Design review of the part built by this model. Coordinates are the model's own, in mm. A direction names the side the tool comes from. Coordinates: 2 decimals unless noted, no trailing zeros. Write each loop counter-clockwise with the first axis right and the second up, starting at its lowest first coordinate (ties: lowest second). Pieces come first, ordered by that corner, then holes. Notation, with made-up numbers: (62, 79.5) - (93, 79.5) arc R6 cw to (93, 88.5) - close; hole circle Ø2 at (49, 23). An arc over 180 degrees is marked (long way). Use a Markdown table: item, result.
from build123d import *

# Parameters (mm, degrees)
BOSS_EXTRUDE1_DEPTH  = 12
BOSS_EXTRUDE11_DEPTH = 12
BOSS_EXTRUDE12_DEPTH = 12
BOSS_EXTRUDE13_DEPTH = 12
SKETCH8_R            = 8
CUT_EXTRUDE1_DEPTH   = 128
SKETCH9_R            = 8
CUT_EXTRUDE2_DEPTH   = 128
SKETCH10_R           = 8
CUT_EXTRUDE4_DEPTH   = 128
FILLET4_R            = 3


with BuildPart() as part:
    # Sketch2 → Boss-Extrude1 (new body)
    with BuildSketch(Plane(origin=(0, 0, 0), x_dir=(1, 0, 0), z_dir=(0, 1, 0))):
        with BuildLine():
            Line((-30, 20), (30, 20))
            ThreePointArc((30, 20), (50, 0), (30, -20))
            Line((30, -20), (-30, -20))
            Line((-30, -20), (-30, 20))
        make_face()
    extrude(amount=BOSS_EXTRUDE1_DEPTH)

    # Sketch3 → Boss-Extrude11 (add)
    with BuildSketch(Plane.XY.offset(20)):
        with BuildLine():
            ThreePointArc((10, 32), (-10, 52), (-30, 32))
            Line((-30, 32), (10, 32))
        make_face()
        with BuildLine():
            ThreePointArc((-30, 32), (-24.142135624, 17.857864376), (-10, 12))
            ThreePointArc((-10, 12), (4.142135624, 17.857864376), (10, 32))
            Line((10, 32), (-30, 32))
        make_face()
        with BuildLine():
            Line((-30, 32), (-30, 12))
            Line((-30, 12), (-10, 12))
            ThreePointArc((-10, 12), (-24.142135624, 17.857864376), (-30, 32))
        make_face()
        with BuildLine():
            ThreePointArc((10, 32), (4.142135624, 17.857864376), (-10, 12))
            Line((-10, 12), (10, 12))
            Line((10, 12), (10, 32))
        make_face()
    extrude(amount=-BOSS_EXTRUDE11_DEPTH)

    # Sketch5 → Boss-Extrude12 (add)
    with BuildSketch(Plane(origin=(0, 0, -20), x_dir=(-1, 0, 0), z_dir=(0, 0, -1))):
        with BuildLine():
            Line((10, 12), (30, 12))
            Line((30, 12), (30, 32))
            ThreePointArc((30, 32), (24.142135624, 17.857864376), (10, 12))
        make_face()
        with BuildLine():
            Line((-10, 12), (10, 12))
            ThreePointArc((10, 12), (-4.142135624, 17.857864376), (-10, 32))
            Line((-10, 32), (-10, 12))
        make_face()
        with BuildLine():
            ThreePointArc((-10, 32), (-4.142135624, 17.857864376), (10, 12))
            ThreePointArc((10, 12), (24.142135624, 17.857864376), (30, 32))
            Line((30, 32), (-10, 32))
        make_face()
        with BuildLine():
            Line((-10, 32), (30, 32))
            ThreePointArc((30, 32), (10, 52), (-10, 32))
        make_face()
    extrude(amount=-BOSS_EXTRUDE12_DEPTH)

    # Sketch6 → Boss-Extrude13 (add)
    with BuildSketch(Plane.ZY.offset(30)):
        with BuildLine():
            Line((20, 0), (0, 0))
            ThreePointArc((0, 0), (14.142135624, -5.857864376), (20, -20))
            Line((20, -20), (20, 0))
        make_face()
        with BuildLine():
            Line((0, 0), (-20, 0))
            Line((-20, 0), (-20, -20))
            ThreePointArc((-20, -20), (-14.142135624, -5.857864376), (0, 0))
        make_face()
        with BuildLine():
            ThreePointArc((20, -20), (14.142135624, -5.857864376), (0, 0))
            ThreePointArc((0, 0), (-14.142135624, -5.857864376), (-20, -20))
            Line((-20, -20), (20, -20))
        make_face()
        with BuildLine():
            Line((20, -20), (-20, -20))
            ThreePointArc((-20, -20), (0, -40), (20, -20))
        make_face()
    extrude(amount=-BOSS_EXTRUDE13_DEPTH)

    # Sketch8 → Cut-Extrude1 (cut)
    with BuildSketch(Plane.XY.offset(20)):
        with Locations((-10, 32)):
            Circle(SKETCH8_R)
    extrude(amount=-CUT_EXTRUDE1_DEPTH, mode=Mode.SUBTRACT)

    # Sketch9 → Cut-Extrude2 (cut)
    with BuildSketch(Plane(origin=(0, 12, 0), x_dir=(1, 0, 0), z_dir=(0, 1, 0))):
        with Locations((30.130515164, -0.017591691)):
            Circle(SKETCH9_R)
    extrude(amount=-CUT_EXTRUDE2_DEPTH, mode=Mode.SUBTRACT)

    # Sketch10 → Cut-Extrude4 (cut)
    with BuildSketch(Plane(origin=(-18, 0, 0), x_dir=(0, 0, -1), z_dir=(1, 0, 0))):
        with Locations((0, -20)):
            Circle(SKETCH10_R)
    extrude(amount=-CUT_EXTRUDE4_DEPTH, mode=Mode.SUBTRACT)

    # Fillet4
    fillet4_edges = [part.edges().sort_by_distance(p)[0] for p in [
        (10, 12, 14),
        (-10, 12, 8),
        (10, 12, -14),
        (-10, 12, -8),
        (-18, 0, 0),
    ]]
    fillet(fillet4_edges, radius=FILLET4_R)


solid = part.part
(1) Take a section at D-D on x = 5. Write out the cut boundary in (y, z), and give its area (3 significant figures).
Determined:
| item | result |
|---|---|
| outline | (0, -20) - (45.23, -20) - (45.23, -8) - (15, -8) arc R3 cw to (12, -5) - (12, 5) arc R3 cw to (15, 8) - (45.23, 8) - (45.23, 20) - (0, 20) - close |
| area | 1,280 mm2 |
(2) For pin 1 (3.5 mm diameter, centred on y = 22.5, z = -15.5, fed in from +X); pin 2 (12 mm diameter, centred on x = 19, z = 5.5, fed in from -Y); pin 3 (6 mm diameter, centred on x = -13.5, y = -18, fed in from +Z); pin 4 (12 mm diameter, centred on x = -9, z = -7, fed in from +Y), all flat-tipped, find the tip position at first contact; note any pin that passes through.
Determined:
| item | result |
|---|---|
| pin 1 | x = 10 |
| pin 2 | y = 0 |
| pin 3 | through |
| pin 4 | y = 52 |
(3) Take a section at A-A on z = -17. Write out the cut boundary in (x, y), and give its area (3 significant figures).
Determined:
| item | result |
|---|---|
| outline | (-30, -30.54) - (-18, -30.54) - (-18, -3) arc R3 cw to (-15, 0) - (40.54, 0) - (40.54, 12) - (13, 12) arc R3 cw to (10, 15) - (10, 32) arc R20 ccw to (-30, 32) - close; hole circle Ø16 at (-10, 32) |
| area | 2,440 mm2 |
(4) For L1, parallel to X at y = 9.5, z = 0.5; L2, parallel to Y at x = -10, z = 11; L3, parallel to X at y = 17, z = 17.5, list the stretches that pass through material, from the lowest coordinate up. Write a range as from..to.
Determined:
| item | result |
|---|---|
| L1 | -30..22.15, 38.12..49.99 |
| L2 | 0..24, 40..52 |
| L3 | -30..10 |
(5) Take a section at B-B on y = 26. Write out the cut boundary in (x, z), and give its area (3 significant figures).
Determined:
| item | result |
|---|---|
| outline | (-30, -20) - (-15.29, -20) - (-15.29, -8) - (-30, -8) - close; (-30, 8) - (-15.29, 8) - (-15.29, 20) - (-30, 20) - close; (-4.71, -20) - (10, -20) - (10, -8) - (-4.71, -8) - close; (-4.71, 8) - (10, 8) - (10, 20) - (-4.71, 20) - close |
| area | 706 mm2 |
(6) Draft analysis for pull direction X (two halves, no side actions). For faces 1 (the cylindrical face through (-11.041, 39.932, -13.916)), 2 (the cylindrical face through (-10, 52, 14)), 3 (the flat face through (19, 12, 0)), state which applies: +X half, -X half, draft (parallel to the pull), parting line (faces both ways), or undercut.
Determined:
| item | result |
|---|---|
| face 1 | undercut |
| face 2 | parting line |
| face 3 | draft |
(7) Take a section at C-C on x = -20.5. Write out the cut boundary in (y, z), and give its area (3 significant figures).
Determined:
| item | result |
|---|---|
| outline | (-20, -20) - (49.02, -20) - (49.02, -8) - (15, -8) arc R3 cw to (12, -5) - (12, 5) arc R3 cw to (15, 8) - (49.02, 8) - (49.02, 20) - (-20, 20) arc R20 ccw to start; hole circle Ø16 at (-20, 0) |
| area | 2,600 mm2 |
(8) Machinability: for faces 4 (the flat face through (18, 0, 0)), 5 (the cylindrical face through (37.76, 6.08, -2.39)), 6 (the cylindrical face through (-8.2, 12.86, 7.1)), 7 (the flat face through (10, 23, 14)), which of the approach directions +Z, -Z, +X, -X, +Y, -Y give a long, thin tool a straight path to every point of the face, cutting with its end or side? Answer none if there is none.
Determined:
| item | result |
|---|---|
| face 4 | +Z, -Z, +X, -Y |
| face 5 | +Y, -Y |
| face 6 | +X, -X, +Y |
| face 7 | +Z, -Z, +X, +Y |
